Build history of the part. All positions in model axes, mm. Face numbers are marked on the shaded views. A direction names the side the tool comes from. Round coordinates to 2 decimals unless told otherwise and drop trailing zeros. Loops run counter-clockwise (first coordinate to the right, second up) from the corner with the lowest first, then second, coordinate; pieces in that order, holes last. Notation, with made-up numbers: (11, 76) - (56, 76) arc R18 ccw to (56, 85) - close; hole circle Ø4 at (49, 9.5). An arc over 180 degrees is marked (long way). One line per question, with ' | ' between items. Start each with the question number.
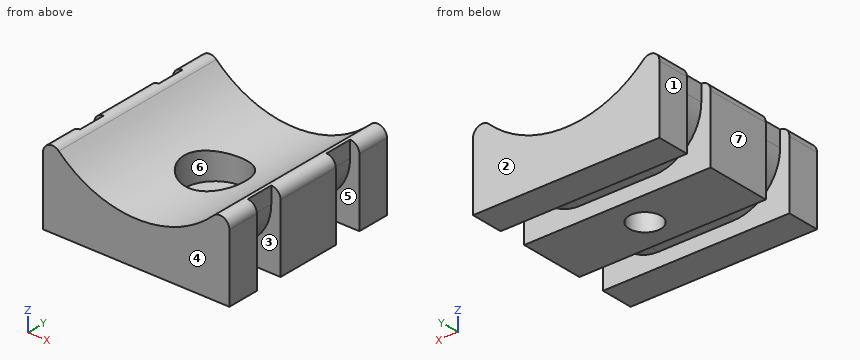
from build123d import *

# Parameters (mm, degrees)
SKETCH_W        = 20
SKETCH_H        = 20
PAD_DEPTH       = 10
SKETCH001_R     = 1.7
POCKET_DEPTH    = 10.001
SKETCH002_R     = 3.3
POCKET001_DEPTH = 8
POCKET002_DEPTH = 20.001
FILLET_R        = 1
SKETCH004_W     = 20
SKETCH004_H     = 3
POCKET003_DEPTH = 1.5
SKETCH005_W     = 3
SKETCH005_H     = 8
POCKET004_DEPTH = 1
SKETCH006_W     = 3
SKETCH006_H     = 8
POCKET005_DEPTH = 1
FILLET001_R     = 5


with BuildPart() as part:
    # Sketch → Pad (new body)
    with BuildSketch(Plane.XY):
        Rectangle(SKETCH_W, SKETCH_H)
    extrude(amount=PAD_DEPTH)

    # Sketch001 → Pocket (cut, through all)
    with BuildSketch(Plane.XY.offset(10)):
        Circle(SKETCH001_R)
    extrude(amount=-POCKET_DEPTH, mode=Mode.SUBTRACT)

    # Sketch002 → Pocket001 (cut)
    with BuildSketch(Plane.XY.offset(10)):
        Circle(SKETCH002_R)
    extrude(amount=-POCKET001_DEPTH, mode=Mode.SUBTRACT)

    # Sketch003 → Pocket002 (cut, through all)
    with BuildSketch(Plane(origin=(0, 10, 0), x_dir=(-1, 0, 0), z_dir=(0, 1, 0))):
        with BuildLine():
            ThreePointArc((-10, 10), (0, 4.63325), (10, 10))
            Line((-10, 10), (10, 10))
        make_face()
    extrude(amount=-POCKET002_DEPTH, mode=Mode.SUBTRACT)

    # Fillet
    fillet_edges = [part.edges().sort_by_distance(p)[0] for p in [
        (-10, 0, 10),
        (10, 0, 10),
    ]]
    fillet(fillet_edges, radius=FILLET_R)

    # Sketch004 → Pocket003 (cut)
    with BuildSketch(Plane(origin=(0, 0, 0), x_dir=(1, 0, 0), z_dir=(0, 0, -1))):
        with Locations((0, 5)):
            Rectangle(SKETCH004_W, SKETCH004_H)
    pocket003 = extrude(amount=-POCKET003_DEPTH, mode=Mode.SUBTRACT)

    # Mirrored: Pocket003 across Sketch004 H_Axis
    add(pocket003.mirror(Plane(origin=(0, 0, 0), x_dir=(0, 0, -1), z_dir=(0, -1, 0))), mode=Mode.SUBTRACT)

    # Sketch005 → Pocket004 (cut)
    with BuildSketch(Plane(origin=(-10, 0, 0), x_dir=(0, -1, 0), z_dir=(-1, 0, 0))):
        with Locations((-5, 5.5)):
            Rectangle(SKETCH005_W, SKETCH005_H)
    pocket004 = extrude(amount=-POCKET004_DEPTH, mode=Mode.SUBTRACT)

    # Mirrored001: Pocket004 across Sketch005 V_Axis
    add(pocket004.mirror(Plane(origin=(-10, 0, 0), x_dir=(-1, 0, 0), z_dir=(0, -1, 0))), mode=Mode.SUBTRACT)

    # Sketch006 → Pocket005 (cut)
    with BuildSketch(Plane.YZ.offset(10)):
        with Locations((-5, 5.5)):
            Rectangle(SKETCH006_W, SKETCH006_H)
    pocket005 = extrude(amount=-POCKET005_DEPTH, mode=Mode.SUBTRACT)

    # Mirrored002: Pocket005 across Sketch006 V_Axis
    add(pocket005.mirror(Plane(origin=(10, 0, 0), x_dir=(1, 0, 0), z_dir=(0, 1, 0))), mode=Mode.SUBTRACT)

    # Fillet001
    fillet001_edges = [part.edges().sort_by_distance(p)[0] for p in [
        (9, 5, 1.5),
        (9, -5, 1.5),
        (-9, -5, 1.5),
        (-9, 5, 1.5),
    ]]
    fillet(fillet001_edges, radius=FILLET001_R)


solid = part.part
1) Saw through at A-A on x = 0. Write the cut outline in (y, z).
2) Saw through at B-B on y = 0. Write the cut outline in (x, z), and give its area (3 significant figures).
3) Drop flat-ended pins along their axis: pin 1 (1.9 mm diameter, centred on y = -5, z = 8, fed in from -X); pin 2 (7.5 mm diameter, centred on x = -0.5, y = 0.5, fed in from +Z); pin 3 (1 mm diameter, centred on x = 2.5, y = -3, fed in from +Z). Give the stop position or say it passes through.
4) Saw through at D-D on z = 6.25. Write the cut outline in (x, y), and give its area (3 significant figures).
5) Saw through at C-C on z = 2.5. Write the cut outline in (x, y).
6) Two-plate mould, pull along Y, no slides. Class the marked faces 1, 2, 3 and 4: +Y half, -Y half, draft (parallel to the pull), parting line (faces both ways), or undercut.
7) Tool access for the marked faces 5, 6 and 7: list every direction of +Z, -Z, +X, -X, +Y, -Y with a clear straight run to the whole face (end or side of a thin tool).
8) Wall check: line 1 (Y direction, x = 0, z = 1.4); line 2 (Y direction, x = 0, z = 2.75); line 3 (Y direction, x = 7, z = 1.75). Give the ranges that are in metal, low to high. Write a range as [from, to].
Answer key:
1) outline: (-10, 0) - (-6.5, 0) - (-6.5, 1.5) - (-3.5, 1.5) - (-3.5, 0) - (-1.7, 0) - (-1.7, 2) - (-3.3, 2) - (-3.3, 4.63) - (-10, 4.63) - close; (1.7, 0) - (3.5, 0) - (3.5, 1.5) - (6.5, 1.5) - (6.5, 0) - (10, 0) - (10, 4.63) - (3.3, 4.63) - (3.3, 2) - (1.7, 2) - close
2) outline: (-10, 0) - (-1.7, 0) - (-1.7, 2) - (-3.3, 2) - (-3.3, 5.1) arc R12 cw to (-8.31, 7.97) arc R1 ccw to (-10, 7.25) - close; (1.7, 0) - (10, 0) - (10, 7.25) arc R1 ccw to (8.31, 7.97) arc R12 cw to (3.3, 5.1) - (3.3, 2) - (1.7, 2) - close | area: 96.5 mm²
3) pin 1: x = -9 | pin 2: z = 5.41 | pin 3: z = 5.01
4) outline: (-10, -10) - (-6.02, -10) - (-6.02, 10) - (-10, 10) - (-10, 6.5) - (-8.99, 6.5) - (-8.99, 3.5) - (-10, 3.5) - (-10, -3.5) - (-8.99, -3.5) - (-8.99, -6.5) - (-10, -6.5) - close; (6.02, -10) - (10, -10) - (10, -6.5) - (8.99, -6.5) - (8.99, -3.5) - (10, -3.5) - (10, 3.5) - (8.99, 3.5) - (8.99, 6.5) - (10, 6.5) - (10, 10) - (6.02, 10) - close | area: 147 mm²
5) outline: (-10, -10) - (10, -10) - (10, -6.5) - (7, -6.5) - (7, -3.5) - (10, -3.5) - (10, 3.5) - (7, 3.5) - (7, 6.5) - (10, 6.5) - (10, 10) - (-10, 10) - (-10, 6.5) - (-7, 6.5) - (-7, 3.5) - (-10, 3.5) - (-10, -3.5) - (-7, -3.5) - (-7, -6.5) - (-10, -6.5) - close; hole circle Ø6.6 at (0, 0)
6) face 1: draft | face 2: +Y half | face 3: undercut | face 4: -Y half
7) face 5: -Z | face 6: +Z | face 7: +Z, -Z, -X, +Y, -Y
8) line 1: [-10, -6.5], [-3.5, -1.7], [1.7, 3.5], [6.5, 10] | line 2: [-10, -3.3], [3.3, 10] | line 3: [-10, -6.5], [-3.5, 3.5], [6.5, 10]
